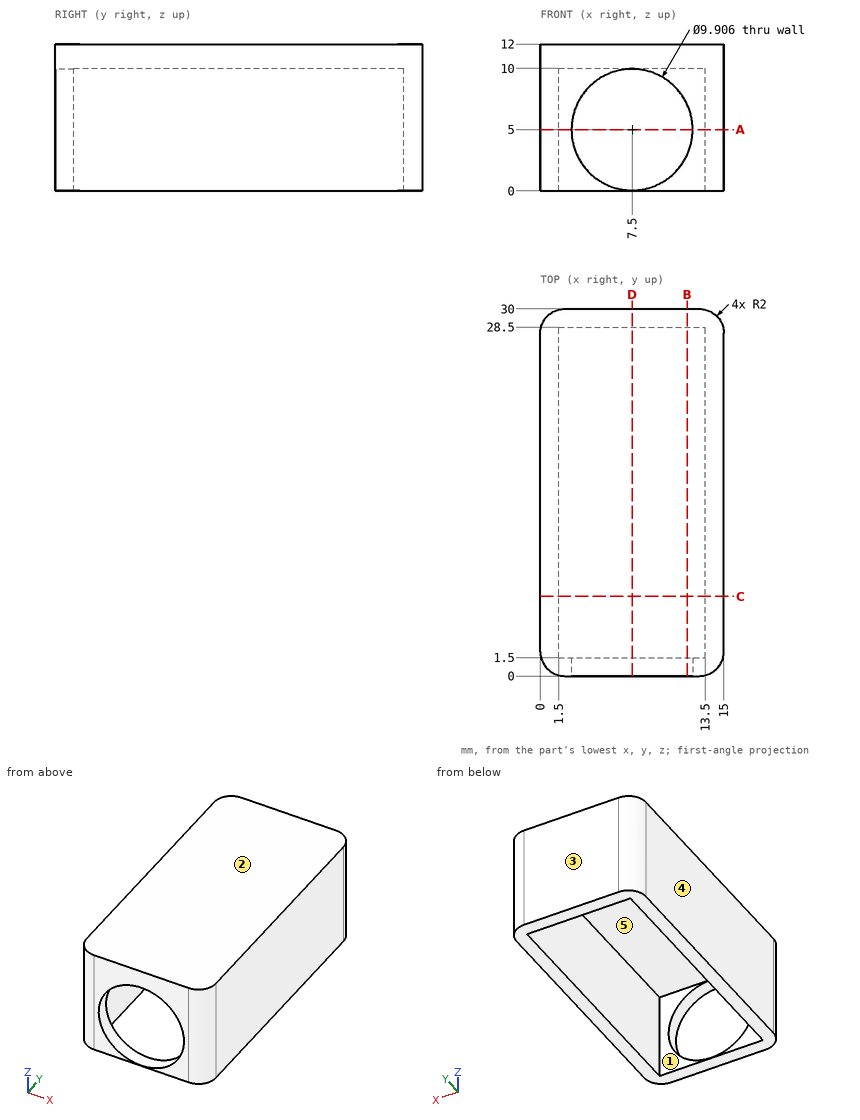
Print and shaded views of the part. All mm, measured from the part's lowest x, y and z. A direction names the side the tool comes from. Coordinates: 2 decimals unless noted, no trailing zeros. Order: outer loops, then holes, each group sorted by start corner. A loop starts at its lowest first (then second) coordinate and runs counter-clockwise, first axis right, second up. Notation, with made-up numbers: (2.5, 80.25) -> (31.5, 80.25) arc R13 cw to (31.5, 100.25) -> close; hole circle Ø8 at (19.25, 58.25). An arc over 180 degrees is marked (long way). Answer as a JSON object with one key per item and string values. Group by question number.
1) Cut at A-A, the plane z = 5. Write the cut outline in (x, y).
2) Pull direction Y, two halves, no side cores. Call the marked faces 3, 4 and 5: +Y half, -Y half, draft (parallel to the pull), parting line (faces both ways), or undercut.
3) Cut at D-D, the plane x = 7.5. Write the cut outline in (y, z).
4) Which spindle directions (+Z, -Z, +X, -X, +Y, -Y) get a long thin tool onto all of the face, cutting with end or side? Do the marked faces 1 and 2. Say none if no direction does.
5) Cut at B-B, the plane x = 12. Write the cut outline in (y, z).
6) Cut at C-C, the plane y = 6.5. Write the cut outline in (x, z).
7) Drill centre lines: L1, parallel to X at y = 7.75, z = 4.5; L2, parallel to Y at x = 2.5, z = 5.75; L3, parallel to Z at x = 11.75, y = 24.5. Where is each one in solid material? Low to high.
8) Flat gauge pins, fed straight in: pin 1 (3 mm diameter, centred on y = 7.5, z = 6, fed in from -X); pin 2 (1 mm diameter, centred on x = 9.5, y = 13.5, fed in from -Z); pin 3 (5 mm diameter, centred on x = 9.5, z = 6, fed in from -Y). Where does each tip first touch, or does it go through?
Check values:
{
 "1": {"outline": "(0, 2) arc R2 ccw to (2, 0) -> (2.55, 0) -> (2.55, 1.5) -> (1.5, 1.5) -> (1.5, 28.5) -> (13.5, 28.5) -> (13.5, 1.5) -> (12.45, 1.5) -> (12.45, 0) -> (13, 0) arc R2 ccw to (15, 2) -> (15, 28) arc R2 ccw to (13, 30) -> (2, 30) arc R2 ccw to (0, 28) -> close"},
 "2": {"face 3": "+Y half", "face 4": "draft", "face 5": "undercut"},
 "3": {"outline": "(0, 0) -> (1.5, 0) -> (1.5, 0.05) -> (0, 0.05) -> close; (0, 9.95) -> (1.5, 9.95) -> (1.5, 10) -> (28.5, 10) -> (28.5, 0) -> (30, 0) -> (30, 12) -> (0, 12) -> close"},
 "4": {"face 1": "-Z", "face 2": "+Z, +X, -X, +Y, -Y"},
 "5": {"outline": "(0, 0) -> (1.5, 0) -> (1.5, 2.93) -> (0, 2.93) -> close; (0, 7.07) -> (1.5, 7.07) -> (1.5, 10) -> (28.5, 10) -> (28.5, 0) -> (30, 0) -> (30, 12) -> (0, 12) -> close"},
 "6": {"outline": "(0, 0) -> (1.5, 0) -> (1.5, 10) -> (13.5, 10) -> (13.5, 0) -> (15, 0) -> (15, 12) -> (0, 12) -> close"},
 "7": {"L1": "x = 0 to 1.5, 13.5 to 15", "L2": "y = 0 to 1.5, 28.5 to 30", "L3": "z = 10 to 12"},
 "8": {"pin 1": "stops at x = 0", "pin 2": "stops at z = 10", "pin 3": "stops at y = 28.5"}
}
